```python
from build123d import *

# Parameters (mm, degrees)
BOX001_W        = 3.5
BOX001_H        = 11
BOX001_DEPTH    = 10
BOX_W           = 6.5
BOX_H           = 5
BOX_DEPTH       = 4
SKETCH010_W     = 10
SKETCH010_H     = 20
PAD004_DEPTH    = 1.2
SKETCH011_R     = 0.7
POCKET004_DEPTH = 1.201
SKETCH012_W     = 10
SKETCH012_H     = 20
PAD005_DEPTH    = 0.2
SKETCH014_W     = 10
SKETCH014_H     = 20
PAD006_DEPTH    = 2
POCKET005_DEPTH = 2
SKETCH015_W     = 10
SKETCH015_H     = 20
PAD007_DEPTH    = 2.5
SKETCH016_R     = 2.2
SKETCH016_W     = 5.8
SKETCH016_H     = 2.7
SKETCH016_W_2   = 2.5
SKETCH016_H_2   = 10.776226
POCKET006_DEPTH = 2.5
FILLET_R        = 3


with BuildPart() as cubo001:
    # Box001 → Box001 (new body)
    with BuildSketch(Plane(origin=(-4, -3, 1), x_dir=(1, 0, 0), z_dir=(0, 0, 1))):
        with Locations((1.75, 5.5)):
            Rectangle(BOX001_W, BOX001_H)
    extrude(amount=BOX001_DEPTH)


with BuildPart() as cubo:
    # Box → Box (new body)
    with BuildSketch(Plane(origin=(-3.5, -10.5, 1), x_dir=(1, 0, 0), z_dir=(0, 0, 1))):
        with Locations((3.25, 2.5)):
            Rectangle(BOX_W, BOX_H)
    extrude(amount=BOX_DEPTH)


with BuildPart() as obj1:
    # Sketch010 → Pad004 (new body)
    with BuildSketch(Plane.XY):
        Rectangle(SKETCH010_W, SKETCH010_H)
    extrude(amount=PAD004_DEPTH)

    # Sketch011 → Pocket004 (cut, through all)
    with BuildSketch(Plane.XY.offset(1.2)):
        with Locations((-1.27, -6.75)):
            Circle(SKETCH011_R)
        with Locations((1.27, -6.75)):
            Circle(SKETCH011_R)
        with Locations((-2, 7.25)):
            Circle(SKETCH011_R)
        with Locations((-2, -1.75)):
            Circle(SKETCH011_R)
        with Locations((2, 4.02)):
            Circle(SKETCH011_R)
        with Locations((2, 1.48)):
            Circle(SKETCH011_R)
    extrude(amount=-POCKET004_DEPTH, mode=Mode.SUBTRACT)

    # Sketch012 → Pad005 (new body)
    with BuildSketch(Plane(origin=(0, 0, 0), x_dir=(1, 0, 0), z_dir=(0, 0, -1))):
        Rectangle(SKETCH012_W, SKETCH012_H)
    extrude(amount=PAD005_DEPTH)

    # Sketch014 → Pad006 (new body)
    with BuildSketch(Plane(origin=(0, 0, -0.2), x_dir=(1, 0, 0), z_dir=(0, 0, -1))):
        Rectangle(SKETCH014_W, SKETCH014_H)
    extrude(amount=PAD006_DEPTH)

    # Sketch013 → Pocket005 (cut)
    with BuildSketch(Plane(origin=(0, 0, -2.2), x_dir=(1, 0, 0), z_dir=(0, 0, -1))):
        Polygon((-3.80896, 8.420167), (3.62375, 8.420167), (3.62375, -5.103398), (0, -7.181223), (0, -8.736001), (-3.696102, -8.736001), (-3.696102, -5.976334), (0.775065, -3.412608), (0.775065, 5.283805), (-0.618984, 5.283805), (-0.618984, 0.458633), (-3.80896, 0.458633), align=None)
    extrude(amount=-POCKET005_DEPTH, mode=Mode.SUBTRACT)

    # Sketch015 → Pad007 (new body)
    with BuildSketch(Plane.XY.offset(1.2)):
        Rectangle(SKETCH015_W, SKETCH015_H)
    extrude(amount=PAD007_DEPTH)

    # Sketch016 → Pocket006 (cut)
    with BuildSketch(Plane.XY.offset(3.7)):
        with Locations((2.024904, 2.79891)):
            Circle(SKETCH016_R)
        with Locations((0, -6.75)):
            Rectangle(SKETCH016_W, SKETCH016_H)
        with Locations((-2.017145, 2.756578)):
            Rectangle(SKETCH016_W_2, SKETCH016_H_2)
    extrude(amount=-POCKET006_DEPTH, mode=Mode.SUBTRACT)

    # Fillet
    fillet_edges = [obj1.edges().sort_by_distance(p)[0] for p in [
        (5, -10, 0.75),
        (-5, -10, 0.75),
        (5, 10, 0.75),
        (-5, 10, 0.75),
    ]]
    fillet(fillet_edges, radius=FILLET_R)

    # Cut: cut Cubo
    add(cubo.part, mode=Mode.SUBTRACT)

    # Cut001: cut Cubo001
    add(cubo001.part, mode=Mode.SUBTRACT)


solid = obj1.part
```
Read the model definition and answer for the solid it produces. Units are mm, in the model's axes. A direction names the side the tool comes from. Give positions to 0.01 mm unless a question says otherwise; leave off trailing zeros. Loops run counter-clockwise (first coordinate to the right, second up) from the corner with the lowest first, then second, coordinate; pieces in that order, holes last.
Item 1: The part is cut by section A-A (z = -1.7). Write down the section's boundary in (x, y).
Item 2: Each of these flat-tipped pins is pushed along its axis until it touches: pin 1 Ø0.8 at (x, z) = (0.5, 3) entering from -Y; pin 2 Ø1.8 at (x, y) = (-1.5, 0.5) entering from +Z; pin 3 Ø0.7 at (x, y) = (2, 1.5) entering from +Z. Where does it stop, or does it pass through?
Item 3: The part is cut by section B-B (y = -6.75). Write down the section's boundary in (x, z).
Item 4: For faces 5 (the flat face through (0, -8, 1)), 6 (the flat face through (-0.5, 2, 2)), 7 (the flat face through (0, -8.42, -1)), determine the directions among +Z, -Z, +X, -X, +Y, -Y from which every point of the face is accessible in a straight line to the end or side of a thin tool.
Item 5: The mould has two halves that part along Y. Classify faces 1 (the flat face through (3, -8, 2)), 2 (the flat face through (0, 10, 1)), 3 (the flat face through (0, -10, -1)), 4 (the flat face through (-1.49, 4.71, -1.21)): released by +Y, released by -Y, zero draft, split by the parting line, or undercut.
Item 6: The part is cut by section C-C (z = 0.8). Write down the section's boundary in (x, y), and give its area (3 significant figures).
Item 7: Find the intervals of material crossed by line 1 along Y through (x, z) = (-2, -1.45); line 2 along X through (y, z) = (-7, 1.7); line 3 along X through (y, z) = (-1.5, -1.3), in increasing order.
Item 8: The part is cut by section D-D (x = 3.25). Write down the section's boundary in (y, z), and give its area (3 significant figures).
Taken from the geometry:
1. outline: (-5, -7) arc R3 ccw to (-2, -10) - (2, -10) arc R3 ccw to (5, -7) - (5, 7) arc R3 ccw to (2, 10) - (-2, 10) arc R3 ccw to (-5, 7) - close; hole (-3.81, -8.42) - (3.62, -8.42) - (3.62, 5.1) - (0, 7.18) - (0, 8.74) - (-3.7, 8.74) - (-3.7, 5.98) - (0.78, 3.41) - (0.78, -5.28) - (-0.62, -5.28) - (-0.62, -0.46) - (-3.81, -0.46) - close
2. pin 1: stops at y = -5.4
2. pin 2: stops at z = 1
2. pin 3: stops at z = 0
3. outline: (-5, -2.2) - (-3.81, -2.2) - (-3.81, -0.2) - (3.62, -0.2) - (3.62, -2.2) - (5, -2.2) - (5, 3.7) - (3, 3.7) - (3, 1) - (1.97, 1) - (1.97, 0) - (0.57, 0) - (0.57, 1) - (-0.57, 1) - (-0.57, 0) - (-1.97, 0) - (-1.97, 1) - (-3.5, 1) - (-3.5, 3.7) - (-5, 3.7) - close
4. face 5: +Z, -Y
4. face 6: +Z
4. face 7: -Z
5. face 1: zero draft
5. face 2: released by +Y
5. face 3: released by -Y
5. face 4: undercut
6. outline: (-5, -7) arc R3 ccw to (-2, -10) - (2, -10) arc R3 ccw to (5, -7) - (5, 7) arc R3 ccw to (2, 10) - (-2, 10) arc R3 ccw to (-5, 7) - close; hole circle Ø1.4 at (-2, -1.75); hole circle Ø1.4 at (-2, 7.25); hole circle Ø1.4 at (-1.27, -6.75); hole circle Ø1.4 at (1.27, -6.75); hole circle Ø1.4 at (2, 1.48); hole circle Ø1.4 at (2, 4.02)
6. area: 183 mm2
7. line 1: y = -10 to -8.42, -0.46 to 5, 8.74 to 10
7. line 2: x = -5 to -3.5, 3 to 5
7. line 3: x = -5 to -3.81, -0.62 to 0.78, 3.62 to 5
8. outline: (-9.73, -2.2) - (-8.42, -2.2) - (-8.42, -0.2) - (5.32, -0.2) - (5.32, -2.2) - (9.73, -2.2) - (9.73, 3.7) - (4.63, 3.7) - (4.63, 1.2) - (0.97, 1.2) - (0.97, 3.7) - (-9.73, 3.7) - close
8. area: 78.2 mm2
